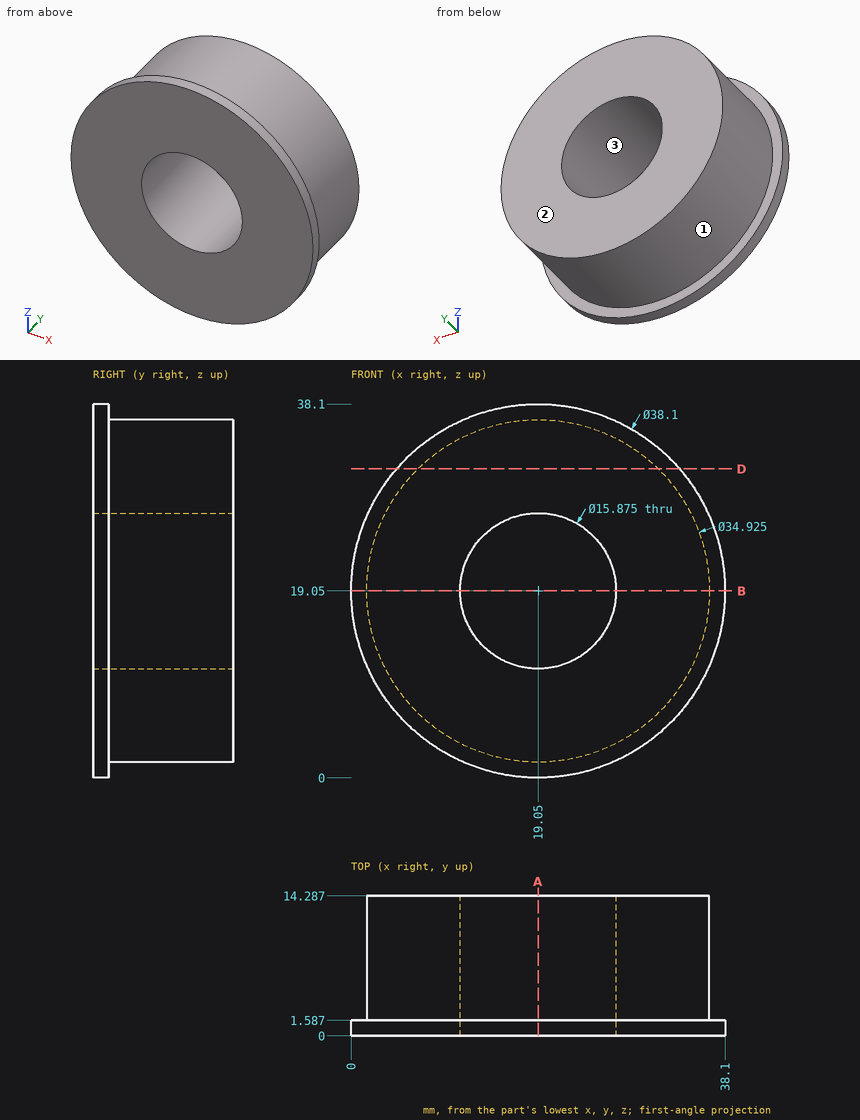
Part print with two shaded views. Sizes in mm from the minimum x, y, z corner. Round coordinates to 2 decimals unless told otherwise and drop trailing zeros. Order: outer loops, then holes, each group sorted by start corner. A loop starts at its lowest first (then second) coordinate and runs counter-clockwise, first axis right, second up. Notation, with made-up numbers: (71, 58.5) - (106, 58.5) arc R17 cw to (106, 84.5) - close; hole circle Ø4 at (-32.75, -16). An arc over 180 degrees is marked (long way). Answer as CSV lines item,"result". Start each with the question number.
1. Drill centre lines: L1, parallel to Z at x = 19.05, y = 5.75; L2, parallel to Z at x = 14.5, y = 6.5 (1 decimal). Where is each one in solid material? Low to high. Write a range as [from, to].
2. Saw through at A-A, the plane x = 19.05. Write the cut outline in (y, z).
3. Saw through at B-B, the plane z = 19.05. Write the cut outline in (x, y), and give its area (3 significant figures).
4. Pull direction Z, two halves, no side cores. Call the marked faces 1, 2 and 3: +Z half, -Z half, draft (parallel to the pull), parting line (faces both ways), or undercut.
5. Pin check, flat tips, straight feed: pin 1 (9.5 mm diameter, centred on x = 19.05, z = 19.05, fed in from +Y); pin 2 (1 mm diameter, centred on x = 22, y = 2.5, fed in from -Z); pin 3 (8 mm diameter, centred on x = 9.5, y = 12, fed in from -Z); pin 4 (1.5 mm diameter, centred on y = 3.5, z = 9.5, fed in from +X). Stop position of each tip, or through.
6. Saw through at D-D, the plane z = 31.5. Write the cut outline in (x, y) (1 decimal).
Model answer:
1,L1,"z = [1.59, 11.11], [26.99, 36.51]"
1,L2,"z = [2.2, 12.5], [25.6, 35.9]"
2,outline,"(0, 0) - (1.59, 0) - (1.59, 1.59) - (14.29, 1.59) - (14.29, 11.11) - (0, 11.11) - close; (0, 26.99) - (14.29, 26.99) - (14.29, 36.51) - (1.59, 36.51) - (1.59, 38.1) - (0, 38.1) - close"
3,outline,"(0, 0) - (11.11, 0) - (11.11, 14.29) - (1.59, 14.29) - (1.59, 1.59) - (0, 1.59) - close; (26.99, 0) - (38.1, 0) - (38.1, 1.59) - (36.51, 1.59) - (36.51, 14.29) - (26.99, 14.29) - close"
3,area,"277 mm²"
4,face 1,"parting line"
4,face 2,"draft"
4,face 3,"undercut"
5,pin 1,"passes through"
5,pin 2,"stops at z = 1.76"
5,pin 3,"stops at z = 2.49"
5,pin 4,"stops at x = 34.13"
6,outline,"(4.6, 0) - (33.5, 0) - (33.5, 1.6) - (31.3, 1.6) - (31.3, 14.3) - (6.8, 14.3) - (6.8, 1.6) - (4.6, 1.6) - close"
